from build123d import *

# Parameters (mm, degrees)
SKETCH1_R           = 7.5
SKETCH1_R_2         = 2.5
BOSS_EXTRUDE1_DEPTH = 10
SKETCH2_R           = 12.7
SKETCH2_R_2         = 2.5
BOSS_EXTRUDE2_DEPTH = 5
SKETCH3_R           = 1.8
CUT_EXTRUDE1_DEPTH  = 16


with BuildPart() as part:
    # Sketch1 → Boss-Extrude1 (new body)
    with BuildSketch(Plane(origin=(0, 0, 0), x_dir=(1, 0, 0), z_dir=(0, 1, 0))):
        Circle(SKETCH1_R)
        Circle(SKETCH1_R_2, mode=Mode.SUBTRACT)
    extrude(amount=BOSS_EXTRUDE1_DEPTH)

    # Sketch2 → Boss-Extrude2 (add)
    with BuildSketch(Plane(origin=(0, 10, 0), x_dir=(-1, 0, 0), z_dir=(0, 1, 0))):
        Circle(SKETCH2_R)
        Circle(SKETCH2_R_2, mode=Mode.SUBTRACT)
    extrude(amount=BOSS_EXTRUDE2_DEPTH)

    # Sketch3 → Cut-Extrude1 (cut, through all)
    with BuildSketch(Plane(origin=(0, 15, 0), x_dir=(-1, 0, 0), z_dir=(0, 1, 0))):
        with Locations((0, -9.525)):
            Circle(SKETCH3_R)
        with Locations((-8.248891971, 4.7625)):
            Circle(SKETCH3_R)
        with Locations((8.248891971, 4.7625)):
            Circle(SKETCH3_R)
    extrude(amount=-CUT_EXTRUDE1_DEPTH, mode=Mode.SUBTRACT)


solid = part.part
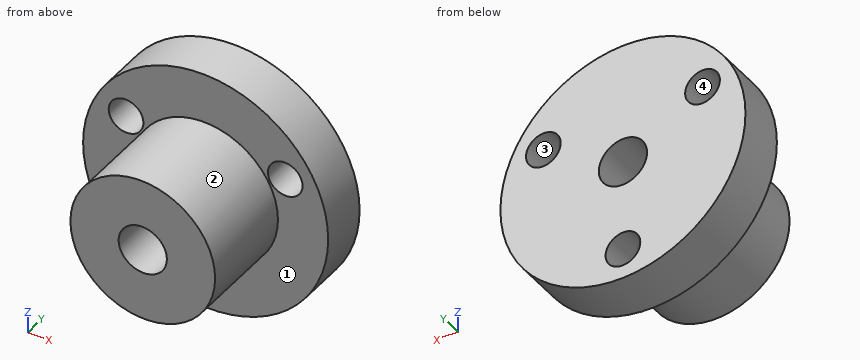
Model file for the job. Use its own axes, mm. Face numbers are marked on the shaded views. Give positions to 0.01 mm unless a question says otherwise; leave off trailing zeros. Loops run counter-clockwise (first coordinate to the right, second up) from the corner with the lowest first, then second, coordinate; pieces in that order, holes last. Notation, with made-up numbers: (57.5, -30) -> (66.5, -30) arc R9 ccw to (66.5, -13) -> close; hole circle Ø2 at (62, 19). An arc over 180 degrees is marked (long way). Use a Markdown table: item, result. Add a question column.
(1) Slice it at D-D on x = -9. List the corners of the cut face in (y, z), and give its area (3 significant figures).
(2) Wall check: line 1 along Z through (x, y) = (0, 13.1) (3 decimals); line 2 along Z through (x, y) = (0, 6). Give the ranges that are in metal, low to high.
(3) Slice it at A-A on x = 0. List the corners of the cut face in (y, z) (3 decimals).
(4) Slice it at B-B on z = 0. List the corners of the cut face in (x, y).
(5) Drop flat-ended pins along their axis: pin 1 Ø1 at (y, z) = (12.5, -2.5) entering from +X; pin 2 Ø3 at (x, z) = (0, 0) entering from -Y; pin 3 Ø8 at (x, y) = (9.5, 5.5) entering from -Z; pin 4 Ø2 at (x, y) = (4, 2) entering from +Z. Give the stop position or say it passes through.
(6) Mould opens along X. For the marked faces 1, 2, 3 and 4 say: +X half, -X half, draft (parallel to the pull), parting line (faces both ways), or undercut.
(7) Slice it at C-C on z = 5.25. List the corners of the cut face in (x, y), and give its area (3 significant figures).
Filled sheet:
| question | item | result |
|---|---|---|
| 1 | outline | (10, -8.96) -> (15, -8.96) -> (15, 3.13) -> (10, 3.13) -> close; (10, 6.4) -> (15, 6.4) -> (15, 8.96) -> (10, 8.96) -> close |
| 1 | area | 73.2 mm2 |
| 2 | line 1 | -12.7 to -11.325, -7.725 to -2.5, 2.5 to 12.7 |
| 2 | line 2 | -7.5 to -2.5, 2.5 to 7.5 |
| 3 | outline | (0, -7.5) -> (10, -7.5) -> (10, -7.725) -> (15, -7.725) -> (15, -2.5) -> (0, -2.5) -> close; (0, 2.5) -> (15, 2.5) -> (15, 12.7) -> (10, 12.7) -> (10, 7.5) -> (0, 7.5) -> close; (10, -12.7) -> (15, -12.7) -> (15, -11.325) -> (10, -11.325) -> close |
| 4 | outline | (-12.7, 10) -> (-7.5, 10) -> (-7.5, 0) -> (-2.5, 0) -> (-2.5, 15) -> (-12.7, 15) -> close; (2.5, 0) -> (7.5, 0) -> (7.5, 10) -> (12.7, 10) -> (12.7, 15) -> (2.5, 15) -> close |
| 5 | pin 1 | x = 12.54 |
| 5 | pin 2 | through |
| 5 | pin 3 | z = -5.1 |
| 5 | pin 4 | z = 6.87 |
| 6 | face 1 | draft |
| 6 | face 2 | parting line |
| 6 | face 3 | undercut |
| 6 | face 4 | undercut |
| 7 | outline | (-11.56, 10) -> (-9.98, 10) -> (-9.98, 15) -> (-11.56, 15) -> close; (-6.52, 10) -> (-5.36, 10) -> (-5.36, 0) -> (5.36, 0) -> (5.36, 10) -> (6.52, 10) -> (6.52, 15) -> (-6.52, 15) -> close; (9.98, 10) -> (11.56, 10) -> (11.56, 15) -> (9.98, 15) -> close |
| 7 | area | 188 mm2 |
